Input: part model. Units: mm. Frame: model coordinates. Face numbers are marked on the shaded views. A direction names the side the tool comes from. Give positions to 0.01 mm unless a question says otherwise; leave off trailing zeros. Order: outer loops, then holes, each group sorted by start corner. A loop starts at its lowest first (then second) coordinate and runs counter-clockwise, first axis right, second up. Notation, with made-up numbers: M 82,67 L 86,67 A14 ccw 86,94 Z; hole C 64.5,62.25 d6. An arc over 180 degrees is marked long. Use a Markdown table: item, result.
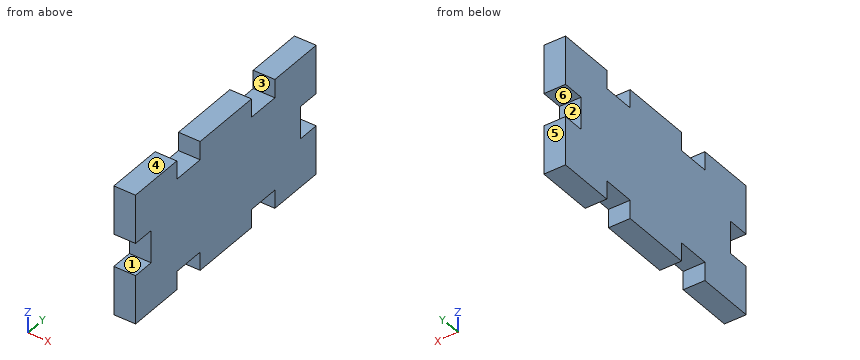
from build123d import *

# Parameters (mm, degrees)
F1_DEPTH = 3.175


with BuildPart() as f1:
    # F0 (on Right) → F1 (new body)
    with BuildSketch(Plane.YZ):
        Polygon((-15.24, 0), (-7.62, 0), (-7.62, 6.819678), (-10.00125, 6.819678), (-10.00125, 9.525), (-18.415, 9.525), (-18.415, 2.38125), (-15.24, 2.38125), align=None)
        Polygon((5.23875, 6.819678), (5.23875, 9.525), (0, 9.525), (0, 0), (7.62, 0), (7.62, 6.819678), align=None)
        Polygon((0, 0), (0, 9.525), (-5.23875, 9.525), (-5.23875, 6.819678), (-7.62, 6.819678), (-7.62, 0), align=None)
        Polygon((18.415, 2.38125), (18.415, 9.525), (10.00125, 9.525), (10.00125, 6.819678), (7.62, 6.819678), (7.62, 0), (15.24, 0), (15.24, 2.38125), align=None)
        Polygon((18.415, -9.525), (18.415, -2.38125), (15.24, -2.38125), (15.24, 0), (7.62, 0), (7.62, -6.819678), (10.00125, -6.819678), (10.00125, -9.525), align=None)
        Polygon((0, -9.525), (0, 0), (-7.62, 0), (-7.62, -6.819678), (-5.23875, -6.819678), (-5.23875, -9.525), align=None)
        Polygon((7.62, -6.819678), (7.62, 0), (0, 0), (0, -9.525), (5.23875, -9.525), (5.23875, -6.819678), align=None)
        Polygon((-7.62, -6.819678), (-7.62, 0), (-15.24, 0), (-15.24, -2.38125), (-18.415, -2.38125), (-18.415, -9.525), (-10.00125, -9.525), (-10.00125, -6.819678), align=None)
    extrude(amount=F1_DEPTH)


solid = f1.part
1) Cut plane B-B on x = 1.7. Return loops of the section in (y, z) (3 decimals).
Response values:
| item | result |
|---|---|
| outline | M -18.415,-9.525 L -10.001,-9.525 L -10.001,-6.82 L -5.239,-6.82 L -5.239,-9.525 L 5.239,-9.525 L 5.239,-6.82 L 10.001,-6.82 L 10.001,-9.525 L 18.415,-9.525 L 18.415,-2.381 L 15.24,-2.381 L 15.24,2.381 L 18.415,2.381 L 18.415,9.525 L 10.001,9.525 L 10.001,6.82 L 5.239,6.82 L 5.239,9.525 L -5.239,9.525 L -5.239,6.82 L -10.001,6.82 L -10.001,9.525 L -18.415,9.525 L -18.415,2.381 L -15.24,2.381 L -15.24,-2.381 L -18.415,-2.381 Z |
2) Cut plane A-A on z = 7.5. Return loops of the section in (x, y) (3 decimals), and give its area (3 significant figures).
Response values:
| item | result |
|---|---|
| outline | M 0,-18.415 L 3.175,-18.415 L 3.175,-10.001 L 0,-10.001 Z; M 0,-5.239 L 3.175,-5.239 L 3.175,5.239 L 0,5.239 Z; M 0,10.001 L 3.175,10.001 L 3.175,18.415 L 0,18.415 Z |
| area | 86.7 mm² |
3) Material intervals for line 1 (Y direction, x = 0.8, z = -7.25) (3 decimals); line 2 (Z direction, x = 1.35, y = -5.5); line 3 (Y direction, x = 0.9, z = -2), sorted ascending. Write a range as from..to.
Response values:
| item | result |
|---|---|
| line 1 | y = -18.415..-10.001, -5.239..5.239, 10.001..18.415 |
| line 2 | z = -6.82..6.82 |
| line 3 | y = -15.24..15.24 |
4) Mould query, pull axis Z, two halves, no side actions, for the marked faces 4, 5 and 6. Classes: released by +Z, released by -Z, zero draft, split by the parting line, or undercut.
Response values:
| item | result |
|---|---|
| face 4 | released by +Z |
| face 5 | zero draft |
| face 6 | undercut |
5) Reachability of the marked faces 1, 2 and 3 from +Z, -Z, +X, -X, +Y, -Y: full face, straight path, thin tool, end or side. Return the list, or none.
Response values:
| item | result |
|---|---|
| face 1 | +X, -X, -Y |
| face 2 | +X, -X, +Y |
| face 3 | +Z, +X, -X |
6) Cut plane C-C on z = -0.75. Return loops of the section in (x, y) (3 decimals), and give its area (3 significant figures).
Response values:
| item | result |
|---|---|
| outline | M 0,-15.24 L 3.175,-15.24 L 3.175,15.24 L 0,15.24 Z |
| area | 96.8 mm² |
7) First-contact query: pin 1 Ø1.6 at (x, y) = (2.5, -7.5) entering from +Z; pin 2 Ø1.6 at (x, y) = (1.5, 6.5) entering from -Z. Flat tips, straight axial feed; report the tip coordinate or a pass-through.
Response values:
| item | result |
|---|---|
| pin 1 | stops at z = 6.82 |
| pin 2 | stops at z = -6.82 |
